The figure shows three views and two pictorial views of one solid part (mm, origin at its lowest corner). Answer the questions. Round coordinates to 2 decimals unless told otherwise and drop trailing zeros. Write each loop counter-clockwise with the first axis right and the second up, starting at its lowest first coordinate (ties: lowest second). Pieces come first, ordered by that corner, then holes. Notation, with made-up numbers: (28.5, -32.75) -> (55.5, -32.75) arc R16 cw to (55.5, -10.75) -> close; hole circle Ø7 at (44.25, -4.5). An arc over 180 degrees is marked (long way). One line per item, written item: value.
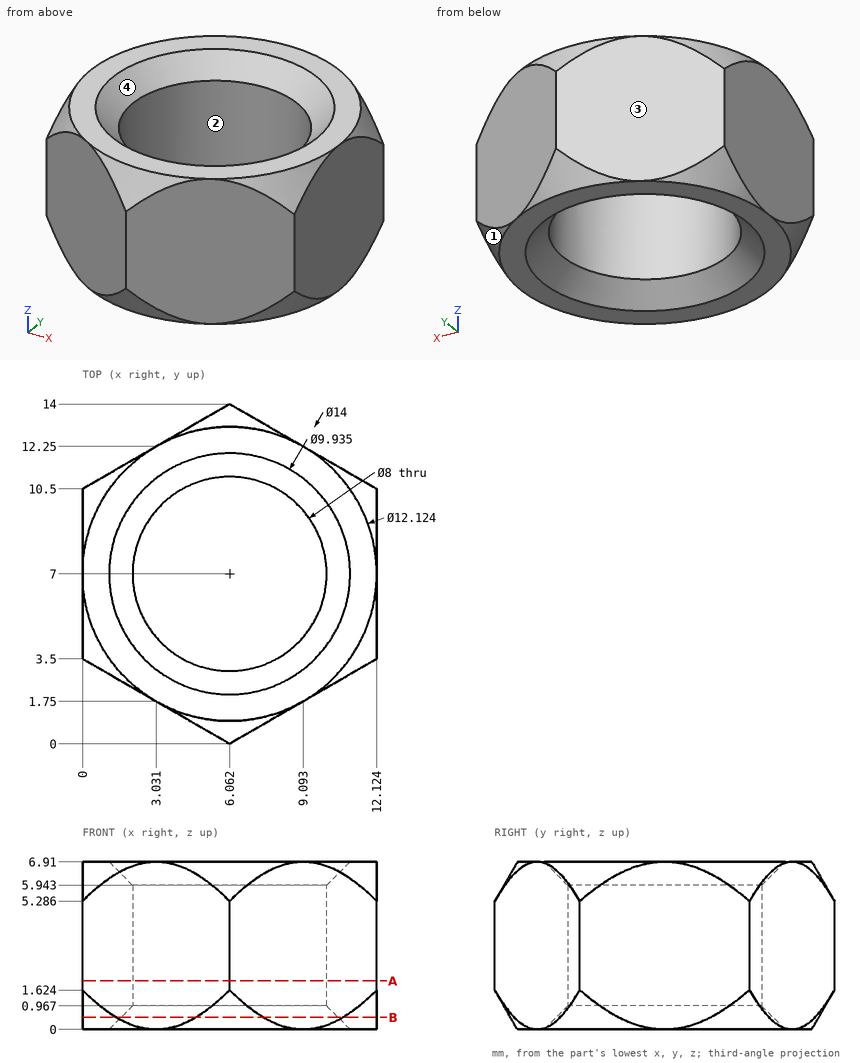
(1) For a pull along X with two mould halves and no side action, classify the marked faces 1, 2, 3 and 4 as pulls with the +X half, pulls with the -X half, needs draft (parallel to the pull), parting line crosses it, or undercut.
Reported:
face 1: pulls with the +X half
face 2: undercut
face 3: pulls with the -X half
face 4: undercut
(2) Consider probe 1 along X at (y, z) = (7.25, 4.75) (1 decimal); probe 2 along Y at (x, z) = (5, 3.75) (1 decimal); probe 3 along Y at (x, z) = (4.5, 6.5). Determine where each line is inside the solid, lowest interval first.
Reported:
probe 1: x = 0 to 2.1, 10.1 to 12.1
probe 2: y = 0.6 to 3.1, 10.9 to 13.4
probe 3: y = 0.9 to 2.72, 11.28 to 13.1
(3) Find section A-A on z = 2. Give the vertices of the cut face in (x, y) (1 decimal).
Reported:
outline: (0, 3.5) -> (6.1, 0) -> (12.1, 3.5) -> (12.1, 10.5) -> (6.1, 14) -> (0, 10.5) -> close; hole circle Ø8 at (6.1, 7)
(4) A flat-ended cylindrical pin translates along its axis: pin 1 Ø3 at (x, z) = (9.5, 3) entering from +Y. Find the tip coordinate at first contact, or state that the pin passes through.
Reported:
pin 1: stops at y = 12.88
(5) Find section B-B on z = 0.5. Give the vertices of the cut face in (x, y) (1 decimal).
Reported:
outline: (0, 5.1) arc R6.4 ccw to (1.4, 2.7) -> (4.7, 0.8) arc R6.4 ccw to (7.5, 0.8) -> (10.7, 2.7) arc R6.4 ccw to (12.1, 5.1) -> (12.1, 8.9) arc R6.4 ccw to (10.7, 11.3) -> (7.5, 13.2) arc R6.4 ccw to (4.7, 13.2) -> (1.4, 11.3) arc R6.4 ccw to (0, 8.9) -> close; hole circle Ø8.9 at (6.1, 7)
